Input: part model. Units: mm. Frame: model coordinates. A direction names the side the tool comes from. Round coordinates to 2 decimals unless told otherwise and drop trailing zeros. Loops run counter-clockwise (first coordinate to the right, second up) from the corner with the lowest first, then second, coordinate; pieces in that order, holes last. Notation, with made-up numbers: M -24.5,-33.75 L 29.5,-33.75 A23 cw 29.5,3.25 Z; hole C -28.5,5.5 d9. An arc over 180 degrees is marked long. Put each result on its own line as item: value. Start each with the question number.
1) Section A-A on x = 0. Output: boundary loops of the cut face in (y, z) (3 decimals).
2) Pin query (flat end, axial travel): pin 1 (2.5 mm diameter, centred on x = 0, y = 0, fed in from +Z). Return the tip coordinate at first contact, or that it passes through.
3) Section C-C on z = 26.5. Output: boundary loops of the cut face in (x, y) (3 decimals).
4) Reachability of faces 3 (the face through (1, -1, 24.32)), 4 (the face through (1, -1, 5.68)), 5 (the face through (0, -1, 15)) from +Z, -Z, +X, -X, +Y, -Y: full face, straight path, thin tool, end or side. Return the list, or none.
5) Line query: probe 1 along Z at (x, y) = (-1, 1.2); probe 2 along Y at (x, z) = (0, 16.25) (3 decimals); probe 3 along Y at (x, z) = (0.45, 15.5). Output: solid intervals per line, ascending.
6) Section B-B on z = 21. Output: boundary loops of the cut face in (x, y) (3 decimals).
7) Draft query along X for faces 1 (the face through (1.49, 2.34, 14.79)), 2 (the face through (2.018, 0.635, 2.88)). Return one class per face: +X half, -X half, draft (parallel to the pull), parting line (faces both ways), or undercut.
from build123d import *

# Parameters (mm, degrees)
SKETCH1_R           = 2.775
BOSS_EXTRUDE1_DEPTH = 30
SKETCH2_R           = 2.27
CUT_EXTRUDE1_DEPTH  = 5.68
CUT_EXTRUDE1_TAPER  = 3.074
SKETCH7_R           = 1
CUT_EXTRUDE2_DEPTH  = 31
SKETCH9_R           = 2.27
CUT_EXTRUDE3_DEPTH  = 5.68
CUT_EXTRUDE3_TAPER  = 3.074


with BuildPart() as part:
    # Sketch1 → Boss-Extrude1 (new body)
    with BuildSketch(Plane.XY):
        Circle(SKETCH1_R)
    extrude(amount=BOSS_EXTRUDE1_DEPTH)

    # Sketch2 → Cut-Extrude1 (cut)
    with BuildSketch(Plane.XY):
        Circle(SKETCH2_R)
    extrude(amount=CUT_EXTRUDE1_DEPTH, taper=CUT_EXTRUDE1_TAPER, mode=Mode.SUBTRACT)

    # Sketch7 → Cut-Extrude2 (cut, through all)
    with BuildSketch(Plane.XY):
        Circle(SKETCH7_R)
    extrude(amount=CUT_EXTRUDE2_DEPTH, mode=Mode.SUBTRACT)

    # Sketch9 → Cut-Extrude3 (cut)
    with BuildSketch(Plane.XY.offset(30)):
        Circle(SKETCH9_R)
    extrude(amount=-CUT_EXTRUDE3_DEPTH, taper=CUT_EXTRUDE3_TAPER, mode=Mode.SUBTRACT)


solid = part.part
Geometry results:
1. outline: M -2.775,0 L -2.27,0 L -1.965,5.68 L -1,5.68 L -1,24.32 L -1.965,24.32 L -2.27,30 L -2.775,30 Z; M 1,5.68 L 1.965,5.68 L 2.27,0 L 2.775,0 L 2.775,30 L 2.27,30 L 1.965,24.32 L 1,24.32 Z
2. pin 1: stops at z = 24.32
3. outline: C 0,0 d5.55; hole C 0,0 d4.164
4. face 3: +Z
4. face 4: -Z
4. face 5: +Z, -Z
5. probe 1: z = 5.68 to 24.32
5. probe 2: y = -2.775 to -1, 1 to 2.775
5. probe 3: y = -2.74 to -0.89, 0.89 to 2.74
6. outline: C 0,0 d5.55; hole C 0,0 d2
7. face 1: parting line
7. face 2: undercut
